The drawing under review shows one solid part. Ordinate dimensions are in mm from its lowest x, y, z. A direction names the side the tool comes from. Coordinates: 2 decimals unless noted, no trailing zeros. Loops run counter-clockwise (first coordinate to the right, second up) from the corner with the lowest first, then second, coordinate; pieces in that order, holes last. Notation, with made-up numbers: (76.25, 18) - (126.25, 18) arc R17 ccw to (126.25, 42) - close; hole circle Ø1 at (52.25, 58.5). An arc over 180 degrees is marked (long way). Answer as a JSON object with one key per item and string values. Group by question number.
Item 1: Tool access review of the marked faces 1 and 2: name each direction out of +Z, -Z, +X, -X, +Y, -Y from which nothing blocks a thin tool from reaching the whole face with its end or side.
Item 2: We need section C-C (y = 5). Give the boundary of the cut face in (x, z), then the cut area to 3 significant figures.
Item 3: We need section D-D (z = 3.25). Give the boundary of the cut face in (x, y).
Item 4: To check wall thickness, follow line 1 (Y direction, x = 16.5, z = 6); line 2 (Z direction, x = 11.75, y = 1.75); line 3 (X direction, y = 12.75, z = 4.75). State the ranges of each line that lie inside material, in increasing order.
Item 5: We need section B-B (x = 3.5). Give the boundary of the cut face in (y, z).
Item 6: We need section A-A (y = 12.5). Give the boundary of the cut face in (x, z), then the cut area to 3 significant figures.
Item 7: Mouldability with a two-part tool opening along Y and no side actions: class the marked faces 3, 4 and 5 as released by +Y, released by -Y, zero draft, split by the parting line, or undercut.
Item 8: Clearance check with a flat-ended pin moving along its axis: pin 1 (2.5 mm diameter, centred on x = 3.5, y = 12.5, fed in from -Z). State where the tip first meets the part, or that it passes through.
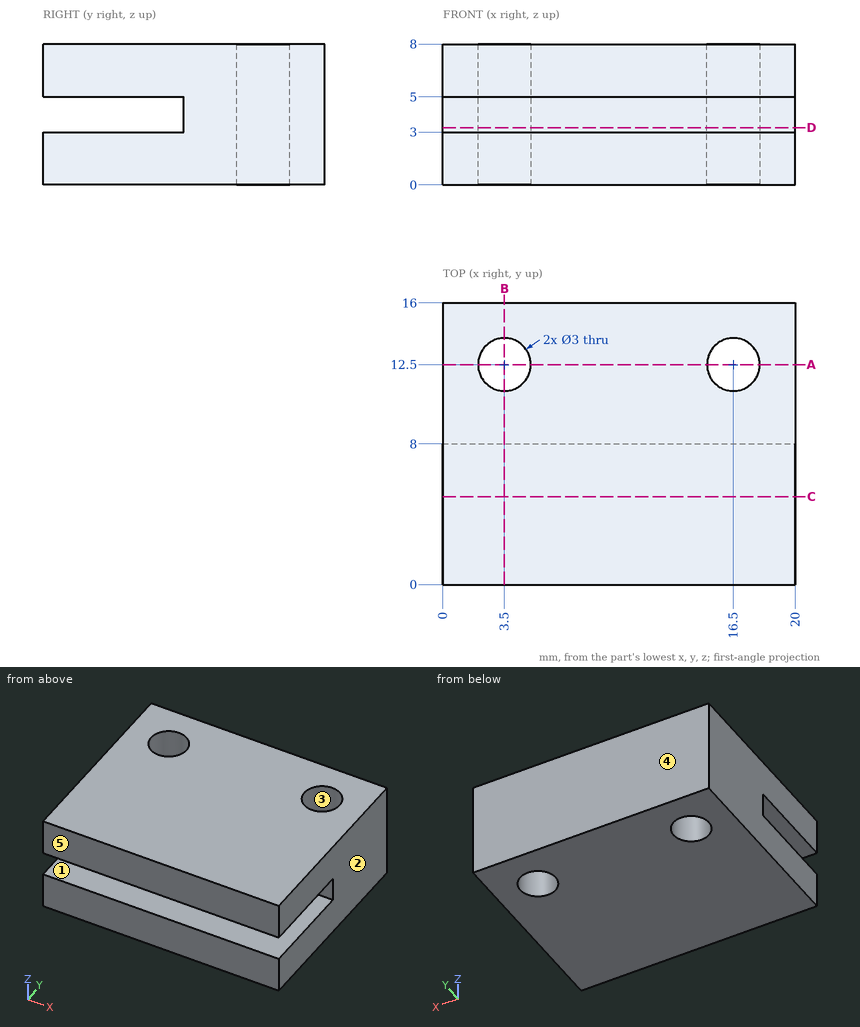
Check sheet entries:
{
 "1": {"face 1": "+X, -X, -Y", "face 2": "+Z, -Z, +X, +Y, -Y"},
 "2": {"outline": "(0, 0) - (20, 0) - (20, 3) - (0, 3) - close; (0, 5) - (20, 5) - (20, 8) - (0, 8) - close", "area": "120 mm2"},
 "3": {"outline": "(0, 8) - (20, 8) - (20, 16) - (0, 16) - close; hole circle Ø3 at (3.5, 12.5); hole circle Ø3 at (16.5, 12.5)"},
 "4": {"line 1": "y = 0 to 11, 14 to 16", "line 2": "z = 0 to 3, 5 to 8", "line 3": "x = 0 to 2.02, 4.98 to 15.02, 17.98 to 20"},
 "5": {"outline": "(0, 0) - (11, 0) - (11, 8) - (0, 8) - (0, 5) - (8, 5) - (8, 3) - (0, 3) - close; (14, 0) - (16, 0) - (16, 8) - (14, 8) - close"},
 "6": {"outline": "(0, 0) - (2, 0) - (2, 8) - (0, 8) - close; (5, 0) - (15, 0) - (15, 8) - (5, 8) - close; (18, 0) - (20, 0) - (20, 8) - (18, 8) - close", "area": "112 mm2"},
 "7": {"face 3": "undercut", "face 4": "released by +Y", "face 5": "released by -Y"},
 "8": {"pin 1": "passes through"}
}
